Geometry: final body of the model. Coordinates: model frame, mm. A direction names the side the tool comes from. Coordinates: 2 decimals unless noted, no trailing zeros. Write each loop counter-clockwise with the first axis right and the second up, starting at its lowest first coordinate (ties: lowest second). Pieces come first, ordered by that corner, then holes. Notation, with made-up numbers: (82.25, -18.75) - (108.25, -18.75) arc R27 cw to (108.25, 2.25) - close; hole circle Ø10 at (36, 84.25). An arc over 180 degrees is marked (long way). Put each result on its own line as item: value.
```python
from build123d import *

# Parameters (mm, degrees)
F1_DEPTH = 38.1
F3_DEPTH = 12.7
F5_DEPTH = 12.7
F7_DEPTH = 25.401


with BuildPart() as f1:
    # F0 (on Front) → F1 (new body)
    with BuildSketch(Plane.XZ):
        Polygon((-7.5456544791, 31.75), (-64.6903658043, 30.9725248881), (-64.6903658043, 0), (-7.5456544791, 0), align=None)
    extrude(amount=F1_DEPTH)

    # F2 (on face) → F3 (cut)
    with BuildSketch(Plane.XZ.offset(38.1)):
        Polygon((-7.5456544791, 31.75), (-45.6421286959, 31.2316832588), (-32.9403658043, 0), (-7.5456544791, 0), align=None)
    extrude(amount=-F3_DEPTH, mode=Mode.SUBTRACT)

    # F4 (on face) → F5 (cut)
    with BuildSketch(Plane(origin=(0, 0, 0), x_dir=(-1, 0, 0), z_dir=(0, 1, 0))):
        Polygon((32.9403658043, 0), (45.6403658043, 31.2317072435), (7.5456544791, 31.75), (7.5456544791, 0), align=None)
    extrude(amount=-F5_DEPTH, mode=Mode.SUBTRACT)

    # F6 (on face) → F7 (cut, through all)
    with BuildSketch(Plane(origin=(0, -12.7, 0), x_dir=(-1, 0, 0), z_dir=(0, 1, 0))):
        Polygon((7.5456544791, 0), (20.2456544791, 31.5772117631), (7.5456544791, 31.75), align=None)
    extrude(amount=-F7_DEPTH, mode=Mode.SUBTRACT)


solid = f1.part
```
1. Section query D-D (z = 4.5). Return loops of the section in (x, y), then the cut area to 3 significant figures.
Answer below:
outline: (-64.69, -38.1) - (-34.77, -38.1) - (-34.77, -25.4) - (-9.36, -25.4) - (-9.36, -12.7) - (-34.77, -12.7) - (-34.77, 0) - (-64.69, 0) - close
area: 1,460 mm²
2. Ray query, probe 1 along Y at (x, z) = (-38.5, 22.5); probe 2 along X at (y, z) = (-14.5, 9.5); probe 3 along Z at (x, y) = (-44.5, -25). Return the intervals inside material, ascending. Write a range as from..to.
Answer below:
probe 1: y = -25.4..-12.7
probe 2: x = -64.69..-11.37
probe 3: z = 0..31.25
3. Pin query (flat end, axial travel): pin 1 Ø1.5 at (x, y) = (-50.5, -19) entering from +Z; pin 2 Ø9.5 at (x, z) = (-19, 8.5) entering from -Y; pin 3 Ø10 at (x, z) = (-22.5, 9) entering from +Y. Return the tip coordinate at first contact, or that it passes through.
Answer below:
pin 1: stops at z = 31.18
pin 2: stops at y = -25.4
pin 3: stops at y = -12.7
4. Set-up query: faces 1 (the flat face through (-26, -12.7, 16)), 2 (the flat face through (-39.38, -31.84, 15.83)), 3 (the flat face through (-53, -38.1, 16)). Return all of +Z, -Z, +X, -X, +Y, -Y with unobstructed straight access to the full face (end or side cutting, diameter ignored); none if empty.
Answer below:
face 1: +Z, +X, +Y
face 2: +Z, +X, -Y
face 3: +Z, -Z, +X, -X, -Y
5. Section query C-C (x = -58). Return loops of the section in (y, z).
Answer below:
outline: (-38.1, 0) - (0, 0) - (0, 31.06) - (-38.1, 31.06) - close
6. Section query A-A (z = 29). Return loops of the section in (x, y), then the cut area to 3 significant figures.
Answer below:
outline: (-64.69, -38.1) - (-44.73, -38.1) - (-44.73, -25.4) - (-19.21, -25.4) - (-19.21, -12.7) - (-44.73, -12.7) - (-44.73, 0) - (-64.69, 0) - close
area: 1,080 mm²
7. Section query B-B (y = -34). Return loops of the section in (x, z), then the cut area to 3 significant figures.
Answer below:
outline: (-64.69, 0) - (-32.94, 0) - (-45.64, 31.23) - (-64.69, 30.97) - close
area: 791 mm²
